from build123d import *

# Parameters (mm, degrees)
SKETCH1_W           = 42.1386
SKETCH1_H           = 42.1386
BOSS_EXTRUDE1_DEPTH = 47.0281
SKETCH2_R           = 10.97915
BOSS_EXTRUDE2_DEPTH = 2.1717
SKETCH3_R           = 2.49555
BOSS_EXTRUDE3_DEPTH = 15.4686
CHAMFER1_SIZE       = 5.08
CHAMFER2_SIZE       = 5.08
CHAMFER3_SIZE       = 5.08
CHAMFER4_SIZE       = 5.08
SKETCH5_R           = 5.588
BOSS_EXTRUDE4_DEPTH = 6.7945


with BuildPart() as part:
    # Sketch1 → Boss-Extrude1 (new body)
    with BuildSketch(Plane(origin=(0, 0, 0), x_dir=(1, 0, 0), z_dir=(0, 1, 0))):
        with Locations((21.0693, 21.0693)):
            Rectangle(SKETCH1_W, SKETCH1_H)
    extrude(amount=BOSS_EXTRUDE1_DEPTH)

    # Sketch2 → Boss-Extrude2 (add)
    with BuildSketch(Plane(origin=(0, 47.0281, 0), x_dir=(1, 0, 0), z_dir=(0, 1, 0))):
        with Locations((21.0693, 21.0693)):
            Circle(SKETCH2_R)
    extrude(amount=BOSS_EXTRUDE2_DEPTH)

    # Sketch3 → Boss-Extrude3 (add)
    with BuildSketch(Plane(origin=(0, 49.1998, 0), x_dir=(1, 0, 0), z_dir=(0, 1, 0))):
        with Locations((21.0693, 21.0693)):
            Circle(SKETCH3_R)
    extrude(amount=BOSS_EXTRUDE3_DEPTH)

    # Chamfer1
    chamfer1_edges = [part.edges().sort_by_distance(p)[0] for p in [
        (42.1386, 23.51405, -42.1386),
    ]]
    chamfer(chamfer1_edges, length=CHAMFER1_SIZE)

    # Chamfer2
    chamfer2_edges = [part.edges().sort_by_distance(p)[0] for p in [
        (42.1386, 23.51405, 0),
    ]]
    chamfer(chamfer2_edges, length=CHAMFER2_SIZE)

    # Chamfer3
    chamfer3_edges = [part.edges().sort_by_distance(p)[0] for p in [
        (0, 23.51405, 0),
    ]]
    chamfer(chamfer3_edges, length=CHAMFER3_SIZE)

    # Chamfer4
    chamfer4_edges = [part.edges().sort_by_distance(p)[0] for p in [
        (0, 23.51405, -42.1386),
    ]]
    chamfer(chamfer4_edges, length=CHAMFER4_SIZE)

    # Sketch5 → Boss-Extrude4 (add)
    with BuildSketch(Plane(origin=(0, 64.6684, 0), x_dir=(1, 0, 0), z_dir=(0, 1, 0))):
        with Locations((21.0693, 21.0693)):
            Circle(SKETCH5_R)
    extrude(amount=BOSS_EXTRUDE4_DEPTH)


solid = part.part
CAD build for the part. Positions are in the model's coordinates, mm. A direction names the side the tool comes from. Give positions to 0.01 mm unless a question says otherwise; leave off trailing zeros. Write each loop counter-clockwise with the first axis right and the second up, starting at its lowest first coordinate (ties: lowest second). Pieces come first, ordered by that corner, then holes. Notation, with made-up numbers: (14.25, 79.25) - (68.25, 79.25) arc R21 ccw to (68.25, 87.25) - close; hole circle Ø11 at (12, 82.25). An arc over 180 degrees is marked (long way). Answer as CSV lines item,"result".
Q1. Band-saw the part on B-B (z = -25). Give the cut face in (x, y).
Result set:
outline,"(0, 0) - (42.14, 0) - (42.14, 47.03) - (31.32, 47.03) - (31.32, 49.2) - (10.82, 49.2) - (10.82, 47.03) - (0, 47.03) - close; (17.1, 64.67) - (25.04, 64.67) - (25.04, 71.46) - (17.1, 71.46) - close"
Q2. Pull direction Y, two halves, no side cores. Call faces 4 (the face through (21, 71.463, -21)), 5 (the face through (21, 0, -21)), 6 (the face through (19.64, 48.099, -31.955)), 7 (the face through (22.23, 64.668, -18.66)): released by +Y, released by -Y, zero draft, split by the parting line, or undercut.
Result set:
face 4,"released by +Y"
face 5,"released by -Y"
face 6,"zero draft"
face 7,"undercut"
Q3. Band-saw the part on A-A (y = 34.5). Give the cut face in (x, z), and give its area (3 significant figures).
Result set:
outline,"(0, -37.06) - (5.08, -42.14) - (37.06, -42.14) - (42.14, -37.06) - (42.14, -5.08) - (37.06, 0) - (5.08, 0) - (0, -5.08) - close"
area,"1,720 mm²"
Q4. Band-saw the part on C-C (x = 9). Give the cut face in (y, z), and give its area (3 significant figures).
Result set:
outline,"(0, -42.14) - (47.03, -42.14) - (47.03, 0) - (0, 0) - close"
area,"1,980 mm²"
Q5. Flat gauge pin, fed straight in: pin 1 Ø6 at (x, z) = (23.5, -5.5) entering from +Y. Where does the tip first touch, or does it go through?
Result set:
pin 1,"y = 47.03"
Q6. 3-axis set-ups, long thin cutter, end or side, ignore diameter. For faces 1 (the face through (20.528, 56.826, -18.633)), 2 (the face through (2.576, 23.185, -39.634)), 3 (the face through (30, 47.028, -12)): which of +Z, -Z, +X, -X, +Y, -Y reach the whole face in a straight line?
Result set:
face 1,"none"
face 2,"-Z, -X, +Y, -Y"
face 3,"+Y"
Q7. Band-saw the part on D-D (z = -29.5). Give the cut face in (x, y).
Result set:
outline,"(0, 0) - (42.14, 0) - (42.14, 47.03) - (28.1, 47.03) - (28.1, 49.2) - (14.04, 49.2) - (14.04, 47.03) - (0, 47.03) - close"
Q8. Drill centre lines: line 1 (Y direction, x = 8.5, z = -19.5); line 2 (Z direction, x = 21, y = 50); line 3 (X direction, y = 7, z = -3). Where is each one in solid material? Low to high. Write a range as from..to.
Result set:
line 1,"0..47.03"
line 2,"-23.56..-18.57"
line 3,"2.08..40.06"
